Check sheet for the drawn part. Datum: minimum x, y, z corner. Units: mm. A direction names the side the tool comes from. Give positions to 0.01 mm unless a question says otherwise; leave off trailing zeros. Loops run counter-clockwise (first coordinate to the right, second up) from the corner with the lowest first, then second, coordinate; pieces in that order, holes last. Notation, with made-up numbers: (26, -30.75) - (75, -30.75) arc R7 ccw to (75, -18.75) - close; hole circle Ø9 at (29.25, -3). An arc over 180 degrees is marked (long way). One line per item, written item: value. Start each with the question number.
1. Mould release check, pull along Z, two halves, no side actions. Record for the marked faces 3, 4 and 5: pulls with the +Z half, pulls with the -Z half, needs draft (parallel to the pull), parting line crosses it, or undercut.
2. Sectioned sample at D-D (y = 40). Record the cut outline in (x, z).
3. Access from +Z, -Z, +X, -X, +Y, -Y to the whole of each face (thin tool, end or side, straight path). Record for the marked faces 1 and 2.
4. Gauge pin test, flat ends, axial feed: pin 1 (1 mm diameter, centred on x = 21.5, z = 114, fed in from +Y); pin 2 (5 mm diameter, centred on y = 16, z = 58.5, fed in from -X); pin 3 (10 mm diameter, centred on y = 31.5, z = 99, fed in from +X). Record the tip position at first contact, or that the pin passes through.
5. Sectioned sample at C-C (z = 72). Record the cut outline in (x, y).
6. Sectioned sample at A-A (z = 25). Record the cut outline in (x, y), plus the area to 3 significant figures.
7. Scan lines: L1, parallel to Z at x = 25, y = 36; L2, parallel to Z at x = 31.5, y = 13.5; L3, parallel to X at y = 47.5, z = 26.5. Record each from-to range of solid material in increasing order. Write a range as [from, to].
8. Sectioned sample at B-B (y = 11.5). Record the cut outline in (x, z).
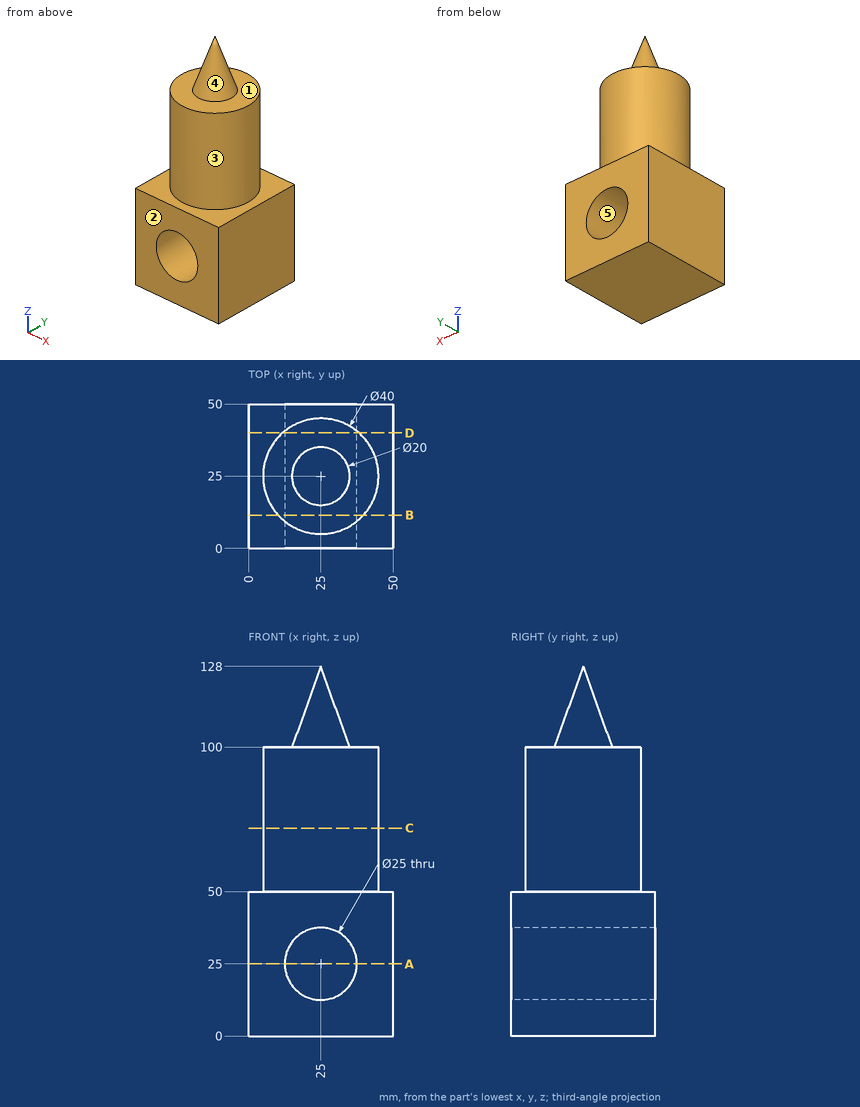
Results are:
1. face 3: needs draft
1. face 4: pulls with the +Z half
1. face 5: undercut
2. outline: (0, 0) - (50, 0) - (50, 50) - (38.23, 50) - (38.23, 100) - (11.77, 100) - (11.77, 50) - (0, 50) - close; hole circle Ø25 at (25, 25)
3. face 1: +Z
3. face 2: +Z, -Z, +X, -X, -Y
4. pin 1: stops at y = 29.06
4. pin 2: stops at x = 6.09
4. pin 3: stops at x = 44.94
5. outline: circle Ø40 at (25, 25)
6. outline: (0, 0) - (12.5, 0) - (12.5, 50) - (0, 50) - close; (37.5, 0) - (50, 0) - (50, 50) - (37.5, 50) - close
6. area: 1,250 mm^2
7. L1: z = [0, 12.5], [37.5, 100]
7. L2: z = [0, 14.32], [35.68, 100]
7. L3: x = [0, 12.59], [37.41, 50]
8. outline: (0, 0) - (50, 0) - (50, 50) - (39.76, 50) - (39.76, 100) - (10.24, 100) - (10.24, 50) - (0, 50) - close; hole circle Ø25 at (25, 25)
